Drawing for the job (mm, zero at the part's lowest x, y, z). A direction names the side the tool comes from. Round coordinates to 2 decimals unless told otherwise and drop trailing zeros. Order: outer loops, then holes, each group sorted by start corner. A loop starts at its lowest first (then second) coordinate and runs counter-clockwise, first axis right, second up. Notation, with made-up numbers: (-28, 18.25) - (5, 18.25) arc R23 cw to (5, 45.25) - close; hole circle Ø10 at (83.25, -22). An arc over 180 degrees is marked (long way). Put each result on its own line as item: value. Start each with the question number.
Item 1: Mould opens along X. For the marked faces 4, 5, 6 and 7 say: pulls with the +X half, pulls with the -X half, needs draft (parallel to the pull), parting line crosses it, or undercut.
Item 2: Saw through at D-D on y = 3. List the corners of the cut face in (x, z).
Item 3: Saw through at B-B on y = 10. List the corners of the cut face in (x, z), plus the area to 3 significant figures.
Item 4: Which spindle directions (+Z, -Z, +X, -X, +Y, -Y) get a long thin tool onto all of the face, cutting with end or side? Do the marked faces 1, 2 and 3. Say none if no direction does.
Item 5: Probe probe 1 along Y at (x, z) = (15, 20.5); probe 2 along Y at (x, z) = (36.5, 13.75); probe 3 along X at (y, z) = (12.5, 19.5). List the from-to ranges inside material, lowest first.
Item 6: Saw through at A-A on x = 21.5. List the corners of the cut face in (y, z).
Item 7: Pin check, flat tips, straight feed: pin 1 Ø3 at (x, z) = (39, 19) entering from -Y; pin 2 Ø9 at (y, z) = (25, 24) entering from +X; pin 3 Ø12.5 at (x, y) = (40, 25.5) entering from +Z. Stop position of each tip, or through.
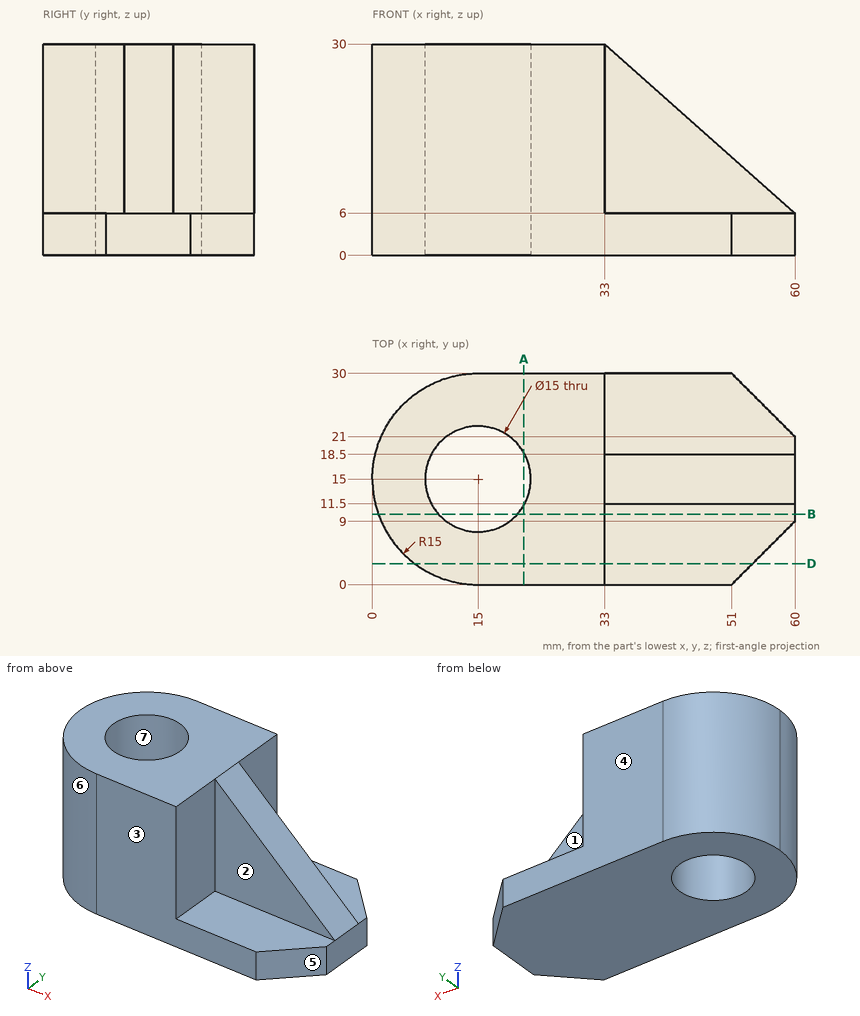
Results found:
1. face 4: needs draft
1. face 5: pulls with the +X half
1. face 6: pulls with the -X half
1. face 7: undercut
2. outline: (6, 0) - (54, 0) - (54, 6) - (33, 6) - (33, 30) - (6, 30) - close
3. outline: (0.86, 0) - (9.41, 0) - (9.41, 30) - (0.86, 30) - close; (20.59, 0) - (60, 0) - (60, 6) - (33, 6) - (33, 30) - (20.59, 30) - close
3. area: 791 mm²
4. face 1: +Z, +X, +Y
4. face 2: +Z, +X, -Y
4. face 3: +Z, -Z, +X, -X, -Y
5. probe 1: y = 0 to 7.5, 22.5 to 30
5. probe 2: y = 11.5 to 18.5
5. probe 3: x = 0.21 to 7.93, 22.07 to 44.81
6. outline: (0, 0) - (11.26, 0) - (11.26, 30) - (0, 30) - close; (18.74, 0) - (30, 0) - (30, 30) - (18.74, 30) - close
7. pin 1: stops at y = 11.5
7. pin 2: stops at x = 33
7. pin 3: stops at z = 6
